Check sheet for the modelled part. Datum: model origin and axes. Units: mm. A direction names the side the tool comes from. Round coordinates to 2 decimals unless told otherwise and drop trailing zeros. Order: outer loops, then holes, each group sorted by start corner. A loop starts at its lowest first (then second) coordinate and runs counter-clockwise, first axis right, second up.
```python
from build123d import *

# Parameters (mm, degrees)
EXTRUDE_1_DEPTH     = 2
SKETCH_4_W          = 11
SKETCH_4_H          = 1.5
EXTRUDE_3_DEPTH     = 4.5
CUT_EXTRUDE_3_DEPTH = 60
SKETCH_6_W          = 1.5
SKETCH_6_H          = 1.5
EXTRUDE_4_DEPTH     = 1.5
SKETCH_8_W          = 1.5
SKETCH_8_H          = 6
EXTRUDE_5_DEPTH     = 4.5
CUT_EXTRUDE_4_DEPTH = 20
SKETCH_12_W         = 1.5
SKETCH_12_H         = 1.5
EXTRUDE_7_DEPTH     = 1.5
SKETCH_13_W         = 1.5
SKETCH_13_H         = 1.5
EXTRUDE_8_DEPTH     = 1.5


with BuildPart() as part:
    # 草图2 → 凸台-拉伸1 (new body)
    with BuildSketch(Plane.XY):
        with BuildLine():
            Line((0, 86.6), (0, 3))
            ThreePointArc((0, 3), (0.878679656, 0.878679656), (3, 0))
            Line((3, 0), (55, 0))
            ThreePointArc((55, 0), (57.121320344, 0.878679656), (58, 3))
            Line((58, 3), (58, 86.6))
            ThreePointArc((58, 86.6), (57.121320344, 88.721320344), (55, 89.6))
            Line((55, 89.6), (3, 89.6))
            ThreePointArc((3, 89.6), (0.878679656, 88.721320344), (0, 86.6))
        make_face()
    extrude(amount=EXTRUDE_1_DEPTH)

    # 草图4 → 凸台-拉伸3 (add)
    with BuildSketch(Plane(origin=(0, 0, 0), x_dir=(-1, 0, 0), z_dir=(0, 0, -1))):
        Polygon((-35, 85.1), (-35, 88.1), (-36.5, 88.1), (-36.5, 86.6), (-47.5, 86.6), (-47.5, 88.1), (-49, 88.1), (-49, 85.1), align=None)
        Polygon((-21.5, 88.1), (-10.5, 88.1), (-9, 88.1), (-9, 85.1), (-23, 85.1), (-23, 88.1), align=None)
        with Locations((-42, 87.35)):
            Rectangle(SKETCH_4_W, SKETCH_4_H)
    extrude(amount=EXTRUDE_3_DEPTH)

    # 草图5 → 切除-拉伸3 (cut)
    with BuildSketch(Plane(origin=(49, 0, 0), x_dir=(0, 0, -1), z_dir=(1, 0, 0))):
        Polygon((1.5, 88.1), (1.5, 86.6), (3, 88.1), align=None)
        Polygon((0, 88.1), (1.5, 86.6), (1.5, 88.1), align=None)
    extrude(amount=-CUT_EXTRUDE_3_DEPTH, mode=Mode.SUBTRACT)

    # 草图6 → 凸台-拉伸4 (add)
    with BuildSketch(Plane(origin=(0, 88.1, 0), x_dir=(1, 0, 0), z_dir=(0, 1, 0))):
        Polygon((9, 0), (10.5, 0), (10.5, 4.5), (9, 4.5), (9, 3), (9, 1.5), align=None)
        Polygon((21.5, 0), (23, 0), (23, 1.5), (23, 3), (23, 4.5), (21.5, 4.5), align=None)
        with Locations((35.75, 3.75)):
            Rectangle(SKETCH_6_W, SKETCH_6_H)
        Polygon((36.5, 3), (35, 3), (35, 1.5), (35, 0), (36.5, 0), align=None)
        Polygon((49, 3), (47.5, 3), (47.5, 0), (49, 0), (49, 1.5), align=None)
        with Locations((48.25, 3.75)):
            Rectangle(SKETCH_6_W, SKETCH_6_H)
    extrude(amount=-EXTRUDE_4_DEPTH)

    # 草图8 → 凸台-拉伸5 (add)
    with BuildSketch(Plane(origin=(0, 0, 0), x_dir=(-1, 0, 0), z_dir=(0, 0, -1))):
        Polygon((-53.5, 24.5), (-56.5, 24.5), (-56.5, 23), (-55, 23), (-55, 17), (-56.5, 17), (-56.5, 15.5), (-53.5, 15.5), align=None)
        with Locations((-55.75, 20)):
            Rectangle(SKETCH_8_W, SKETCH_8_H)
        Polygon((-4.5, 15.5), (-4.5, 24.5), (-1.5, 24.5), (-1.5, 23), (-1.5, 17), (-1.5, 15.5), align=None)
    extrude(amount=EXTRUDE_5_DEPTH)

    # 草图9 → 切除-拉伸4 (cut)
    with BuildSketch(Plane.XZ.offset(-15.5)):
        Polygon((1.5, -3), (3, -1.5), (1.5, 0), align=None)
        Polygon((56.5, -3), (56.5, 0), (55, -1.5), align=None)
    extrude(amount=-CUT_EXTRUDE_4_DEPTH, mode=Mode.SUBTRACT)

    # 草图12 → 凸台-拉伸7 (add)
    with BuildSketch(Plane.ZY.offset(-1.5)):
        Polygon((0, 23), (0, 24.5), (-1.5, 24.5), (-3, 24.5), (-3, 23), align=None)
        Polygon((0, 15.5), (0, 17), (-3, 17), (-3, 15.5), (-1.5, 15.5), align=None)
        with Locations((-3.75, 23.75)):
            Rectangle(SKETCH_12_W, SKETCH_12_H)
        with Locations((-3.75, 16.25)):
            Rectangle(SKETCH_12_W, SKETCH_12_H)
    extrude(amount=-EXTRUDE_7_DEPTH)

    # 草图13 → 凸台-拉伸8 (add)
    with BuildSketch(Plane(origin=(56.5, 0, 0), x_dir=(0, 0, -1), z_dir=(1, 0, 0))):
        with Locations((3.75, 16.25)):
            Rectangle(SKETCH_13_W, SKETCH_13_H)
        Polygon((3, 17), (0, 17), (0, 15.5), (1.5, 15.5), (3, 15.5), align=None)
        with Locations((3.75, 23.75)):
            Rectangle(SKETCH_13_W, SKETCH_13_H)
        Polygon((1.5, 24.5), (0, 24.5), (0, 23), (3, 23), (3, 24.5), align=None)
    extrude(amount=-EXTRUDE_8_DEPTH)


solid = part.part
```
Item 1: Scan lines: line 1 along Z through (x, y) = (24, 24.5); line 2 along X through (y, z) = (21, -1.5); line 3 along Y through (x, z) = (40.5, -3.25). Record each from-to range of solid material in increasing order.
Answer:
line 1: z = 0 to 2
line 2: x = 3 to 4.5, 53.5 to 55
line 3: y = 85.1 to 88.1
Item 2: Release check for a two-part mould opening along X. For faces 1 (the flat face through (29, 45, 2)), 2 (the flat face through (53.5, 20, -2)), 3 (the cylindrical face through (0.86, 0.9, 0.99)) record: released by +X, released by -X, zero draft, split by the parting line, or undercut.
Answer:
face 1: zero draft
face 2: undercut
face 3: released by -X
Item 3: Access from +Z, -Z, +X, -X, +Y, -Y to the whole of each face (thin tool, end or side, straight path). Record for faces 4 (the flat face through (16, 85.1, -2)), 5 (the flat face through (41.9, 88.1, -3.3)), 6 (the flat face through (9, 87, -2)).
Answer:
face 4: -Z, +X, -X, -Y
face 5: -Z, +X, -X, +Y
face 6: -Z, -X, +Y, -Y
Item 4: Sectioned sample at A-A (x = 19). Record the cut outline in (y, z), and give its area (3 significant figures).
Answer:
outline: (0, 0) - (85.1, 0) - (85.1, -4.5) - (88.1, -4.5) - (88.1, -3) - (86.6, -1.5) - (88.1, 0) - (89.6, 0) - (89.6, 2) - (0, 2) - close
area: 190 mm2
Item 5: Go/stop test with flat-tipped pins: P1, Ø2, axis at y = 18, z = -3, coming from the +X side; P2, Ø1.2, axis at x = 56, z = -1.5, coming from the -Y side; P3, Ø1.5, axis at x = 35.5, z = -3.5, coming from the -Y side. Record where each tip stops, or that it passes through.
Answer:
P1: stops at x = 56.5
P2: stops at y = 15.5
P3: stops at y = 85.1
Item 6: Sectioned sample at C-C (x = 34). Record the cut outline in (y, z).
Answer:
outline: (0, 0) - (89.6, 0) - (89.6, 2) - (0, 2) - close
Item 7: Sectioned sample at B-B (y = 13). Record the cut outline in (x, z).
Answer:
outline: (0, 0) - (58, 0) - (58, 2) - (0, 2) - close
